Input: part model. Units: mm. Frame: model coordinates. Face numbers are marked on the shaded views. A direction names the side the tool comes from. Coordinates: 2 decimals unless noted, no trailing zeros. Loops run counter-clockwise (first coordinate to the right, second up) from the corner with the lowest first, then second, coordinate; pieces in that order, holes last. Notation, with made-up numbers: M 31,86 L 74,86 A33 cw 74,125 Z; hole C 29.5,37.25 d6. An arc over 180 degrees is marked long. Use a Markdown table: item, result. Add a question column.
1. Section D-D on x = -96.5. Output: boundary loops of the cut face in (y, z), then the cut area to 3 significant figures.
2. Section C-C on y = -2. Output: boundary loops of the cut face in (x, z), then the cut area to 3 significant figures.
3. Pin query (flat end, axial travel): pin 1 (4 mm diameter, centred on y = -4, z = -7, fed in from +X); pin 2 (5 mm diameter, centred on x = 43, z = 4, fed in from +Y); pin 3 (3 mm diameter, centred on x = 40.5, y = -0.5, fed in from +Z). Return the tip coordinate at first contact, or that it passes through.
4. Line query: L1, parallel to X at y = -0.25, z = -5.5; L2, parallel to Z at x = -36, y = 7.75; L3, parallel to Z at x = -33, y = 7. Output: solid intervals per line, ascending. Write a range as [from, to].
5. Section A-A on z = 0. Output: boundary loops of the cut face in (x, y).
6. Set-up query: the marked faces 1, 2 and 3. Return all of +Z, -Z, +X, -X, +Y, -Y with unobstructed straight access to the full face (end or side cutting, diameter ignored); none if empty.
7. Section B-B on x = -50.5. Output: boundary loops of the cut face in (y, z).
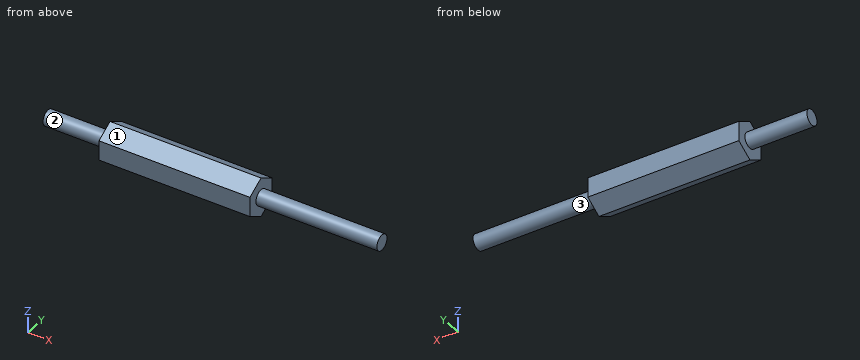
```python
from build123d import *

# Parameters (mm, degrees)
F1_DEPTH = 77.3176
F2_R     = 3.9624
F3_DEPTH = 31.75
F4_R     = 3.96875
F5_DEPTH = 61.8998


with BuildPart() as f1:
    # F0 (on Right) → F1 (new body)
    with BuildSketch(Plane.YZ):
        Polygon((8.7122, -5.029991), (8.7122, 5.029991), (0, 10.059982), (-8.7122, 5.029991), (-8.7122, -5.029991), (0, -10.059982), align=None)
    extrude(amount=-F1_DEPTH)

    # F2 (on face) → F3 (join)
    with BuildSketch(Plane(origin=(-77.3176, 0, 0), x_dir=(0, -1, 0), z_dir=(-1, 0, 0))):
        Circle(F2_R)
    extrude(amount=F3_DEPTH)

    # F4 (on face) → F5 (join)
    with BuildSketch(Plane.YZ):
        Circle(F4_R)
    extrude(amount=F5_DEPTH)


solid = f1.part
```
Answers below:
| question | item | result |
|---|---|---|
| 1 | outline | C 0,0 d7.92 |
| 1 | area | 49.3 mm² |
| 2 | outline | M -109.07,-3.42 L -77.32,-3.42 L -77.32,-8.91 L 0,-8.91 L 0,-3.43 L 61.9,-3.43 L 61.9,3.43 L 0,3.43 L 0,8.91 L -77.32,8.91 L -77.32,3.42 L -109.07,3.42 Z |
| 2 | area | 2,020 mm² |
| 3 | pin 1 | stops at x = 0 |
| 3 | pin 2 | stops at y = 3.67 |
| 3 | pin 3 | stops at z = 3.97 |
| 4 | L1 | x = [-77.32, 0] |
| 4 | L2 | z = [-5.59, 5.59] |
| 4 | L3 | z = [-6.02, 6.02] |
| 5 | outline | M -109.07,-3.96 L -77.32,-3.96 L -77.32,-8.71 L 0,-8.71 L 0,-3.97 L 61.9,-3.97 L 61.9,3.97 L 0,3.97 L 0,8.71 L -77.32,8.71 L -77.32,3.96 L -109.07,3.96 Z |
| 6 | face 1 | +Z, +X, -X, -Y |
| 6 | face 2 | -X |
| 6 | face 3 | +X |
| 7 | outline | M -8.71,-5.03 L 0,-10.06 L 8.71,-5.03 L 8.71,5.03 L 0,10.06 L -8.71,5.03 Z |
